For this review, take the finished solid that the model builds, in its own axes (mm). A direction names the side the tool comes from. Coordinates: 2 decimals unless noted, no trailing zeros. Loops run counter-clockwise (first coordinate to the right, second up) from the corner with the lowest first, then second, coordinate; pieces in that order, holes last. Notation, with made-up numbers: M 14,-14 L 67,-14 A9 ccw 67,-5 Z; hole C 52,-20 d3. An arc over 180 degrees is marked long. Answer as a JSON object with one key per item and string values. Group by question number.
Item 1: Add section C-C (z = -46). State the section outline as (x, y) points.
Item 2: Tool access review of faces 1 (the face through (89, 2, -21)), 2 (the face through (22, 5, -29)), 3 (the face through (133.797, 4.93, -19.141)): name each direction out of +Z, -Z, +X, -X, +Y, -Y from which nothing blocks a thin tool from reaching the whole face with its end or side.
Item 3: Insertion check: pin 1 (5 mm diameter, centred on y = 6, z = -27, fed in from +X); pin 2 (2.5 mm diameter, centred on y = 2.5, z = -27.5, fed in from +X); pin 3 (5 mm diameter, centred on x = 74, y = 7, fed in from +Z). Each pin has a flat end and moves straight along its axis. Give the tip position at first contact, or say it passes through.
Item 4: Add section D-D (x = 35). State the section outline as (y, z) points, then the cut area to 3 significant figures.
Item 5: Wall thickness on L1, parallel to X at y = 4.25, z = -10; L2, parallel to X at y = 1.5, z = -24.5; L3, parallel to X at y = 7.5, z = -26: over which ranges is each line inside the solid? List them lowest first. Write a range as from..to.
Item 6: Mouldability with a two-part tool opening along X and no side actions: class faces 4 (the face through (150.678, 4.93, -21.927)), 5 (the face through (49.11, 4.93, -31.84)), 6 (the face through (97, 5, -28)), 7 (the face through (161.4, 4.9, -9)) as +X half, -X half, draft (parallel to the pull), parting line (faces both ways), or undercut.
Item 7: Add section A-A (x = 145). State the section outline as (y, z) points, then the cut area to 3 significant figures.
Item 8: Add section B-B (x = 74). State the section outline as (y, z) points.
from build123d import *

# Parameters (mm, degrees)
SKETCH1_R           = 2.6
SKETCH1_R_2         = 2.1
SKETCH1_R_3         = 4.2
SKETCH1_R_4         = 2.5
BOSS_EXTRUDE1_DEPTH = 10
FILLET2_R           = 6
FILLET3_R           = 3
CUT_EXTRUDE1_DEPTH  = 11
SKETCH7_R           = 2.6
CUT_EXTRUDE4_DEPTH  = 11
FILLET8_R           = 5
FILLET9_R           = 4
SKETCH10_W          = 34
SKETCH10_H          = 10
CUT_EXTRUDE6_DEPTH  = 11
FILLET10_R          = 4
CUT_EXTRUDE7_DEPTH  = 5
FILLET14_R          = 6
FILLET15_R          = 2
FILLET16_R          = 10
FILLET17_R          = 8
FILLET18_R          = 4


with BuildPart() as part:
    # Sketch1 → Boss-Extrude1 (new body)
    with BuildSketch(Plane(origin=(0, 0, 0), x_dir=(1, 0, 0), z_dir=(0, 1, 0))):
        Polygon((164, 15), (139, 28), (92, 28), (87, 32), (17, 50), (18, 84), (11, 84), (1, 51), (-8, 22), (-14, 14), (-14, 2), (-14, -1), (-6, -1), (0, 0), (139, 0), (164, 3), align=None)
        with Locations((-7, 10)):
            Circle(SKETCH1_R, mode=Mode.SUBTRACT)
        with Locations((159, 10)):
            Circle(SKETCH1_R, mode=Mode.SUBTRACT)
        with Locations((5, 26)):
            Circle(SKETCH1_R_2, mode=Mode.SUBTRACT)
        with Locations((9, 40)):
            Circle(SKETCH1_R_3, mode=Mode.SUBTRACT)
        with Locations((145, 13)):
            Circle(SKETCH1_R_4, mode=Mode.SUBTRACT)
    extrude(amount=BOSS_EXTRUDE1_DEPTH)

    # Fillet2
    fillet2_edges = [part.edges().sort_by_distance(p)[0] for p in [
        (139, 5, -28),
        (164, 5, -15),
        (164, 5, -3),
    ]]
    fillet(fillet2_edges, radius=FILLET2_R)

    # Fillet3
    fillet3_edges = [part.edges().sort_by_distance(p)[0] for p in [
        (11, 5, -84),
        (18, 5, -84),
    ]]
    fillet(fillet3_edges, radius=FILLET3_R)

    # Sketch4 → Cut-Extrude1 (cut, through all)
    with BuildSketch(Plane(origin=(0, 10, 0), x_dir=(1, 0, 0), z_dir=(0, 1, 0))):
        Polygon((22, 39), (22, 20), (50, 20), (50, 32.5), align=None)
    extrude(amount=-CUT_EXTRUDE1_DEPTH, mode=Mode.SUBTRACT)

    # Sketch7 → Cut-Extrude4 (cut, through all)
    with BuildSketch(Plane(origin=(0, 10, 0), x_dir=(1, 0, 0), z_dir=(0, 1, 0))):
        with Locations((47, 6)):
            Circle(SKETCH7_R)
    extrude(amount=-CUT_EXTRUDE4_DEPTH, mode=Mode.SUBTRACT)

    # Fillet8
    fillet8_edges = [part.edges().sort_by_distance(p)[0] for p in [
        (-14, 5, 1),
    ]]
    fillet(fillet8_edges, radius=FILLET8_R)

    # Fillet9
    fillet9_edges = [part.edges().sort_by_distance(p)[0] for p in [
        (22, 5, -39),
        (50, 5, -32.5),
        (50, 5, -20),
        (22, 5, -20),
    ]]
    fillet(fillet9_edges, radius=FILLET9_R)

    # Sketch10 → Cut-Extrude6 (cut, through all)
    with BuildSketch(Plane(origin=(0, 10, 0), x_dir=(1, 0, 0), z_dir=(0, 1, 0))):
        with Locations((118, 23)):
            Rectangle(SKETCH10_W, SKETCH10_H)
    extrude(amount=-CUT_EXTRUDE6_DEPTH, mode=Mode.SUBTRACT)

    # Fillet10
    fillet10_edges = [part.edges().sort_by_distance(p)[0] for p in [
        (135, 5, -18),
        (101, 5, -18),
    ]]
    fillet(fillet10_edges, radius=FILLET10_R)

    # Sketch12 → Cut-Extrude7 (cut)
    with BuildSketch(Plane(origin=(0, 0, 0), x_dir=(1, 0, 0), z_dir=(0, 1, 0))):
        Polygon((58, 37), (83, 31.034746853), (89, 26.034746853), (89, 14), (58, 14), align=None)
    extrude(amount=CUT_EXTRUDE7_DEPTH, mode=Mode.SUBTRACT)

    # Fillet14
    fillet14_edges = [part.edges().sort_by_distance(p)[0] for p in [
        (87, 5, -32),
        (92, 5, -28),
    ]]
    fillet(fillet14_edges, radius=FILLET14_R)

    # Fillet15
    fillet15_edges = [part.edges().sort_by_distance(p)[0] for p in [
        (101, 5, -28),
        (135, 5, -28),
    ]]
    fillet(fillet15_edges, radius=FILLET15_R)

    # Fillet16
    fillet16_edges = [part.edges().sort_by_distance(p)[0] for p in [
        (17, 5, -50),
    ]]
    fillet(fillet16_edges, radius=FILLET16_R)

    # Fillet17
    fillet17_edges = [part.edges().sort_by_distance(p)[0] for p in [
        (-14, 5, -14),
        (-8, 5, -22),
    ]]
    fillet(fillet17_edges, radius=FILLET17_R)

    # Fillet18
    fillet18_edges = [part.edges().sort_by_distance(p)[0] for p in [
        (58, 2.5, -37),
        (58, 2.5, -14),
        (89, 2.5, -14),
        (89, 2.5, -26.034746853),
        (83, 2.5, -31.034746853),
    ]]
    fillet(fillet18_edges, radius=FILLET18_R)


solid = part.part
From the geometry:
{
 "1": {"outline": "M -0.55,0 L 32.56,0 L 32.56,10 L -0.55,10 Z"},
 "2": {"face 1": "-Y", "face 2": "+Y, -Y", "face 3": "-Z, +Y, -Y"},
 "3": {"pin 1": "stops at x = 145.73", "pin 2": "stops at x = 142.37", "pin 3": "stops at z = 0"},
 "4": {"outline": "M 0,-45.37 L 10,-45.37 L 10,-35.98 L 0,-35.98 Z; M 0,-20 L 10,-20 L 10,0 L 0,0 Z", "area": "294 mm²"},
 "5": {"L1": "x = -14..-9.6, -4.4..156.4, 161.6..164", "L2": "x = -7.22..3.53, 6.47..22, 50..58, 88.99..101, 135..145.73", "L3": "x = -6.76..2.9, 7.1..22, 50..101, 135..142.85"},
 "6": {"face 4": "+X half", "face 5": "undercut", "face 6": "draft", "face 7": "undercut"},
 "7": {"outline": "M 0,-24.88 L 10,-24.88 L 10,-15.5 L 0,-15.5 Z; M 0,-10.5 L 10,-10.5 L 10,-0.72 L 0,-0.72 Z", "area": "192 mm²"},
 "8": {"outline": "M 0,-35.34 L 10,-35.34 L 10,0 L 0,0 L 0,-14 L 5,-14 L 5,-33.18 L 0,-33.18 Z"}
}
